```python
from build123d import *

# Parameters (mm, degrees)
BOSS_EXTRUDE1_DEPTH   = 9.525
FILLET1_R             = 5.08
F_5_0MM_DOWEL_HOLE1_D = 5
SKETCH14_R            = 2.5
CUT_EXTRUDE1_DEPTH    = 139.21913576


with BuildPart() as part:
    # Sketch1 → Boss-Extrude1 (new body)
    with BuildSketch(Plane.XY):
        Polygon((-27.510468203, 50), (27.510468203, 50), (67.924987047, 120), (67.924987047, 81.9), (20.64, 0), (10, -99.432340815), (-10, -99.432340815), (-20.64, 0), (-67.924987047, 81.9), (-67.924987047, 120), align=None)
    extrude(amount=BOSS_EXTRUDE1_DEPTH)

    # Fillet1
    fillet1_edges = [part.edges().sort_by_distance(p)[0] for p in [
        (-27.510468203, 50, 4.7625),
        (27.510468203, 50, 4.7625),
        (67.924987047, 81.9, 4.7625),
        (20.64, 0, 4.7625),
        (10, -99.432340815, 4.7625),
        (-10, -99.432340815, 4.7625),
        (-20.64, 0, 4.7625),
        (-67.924987047, 81.9, 4.7625),
    ]]
    fillet(fillet1_edges, radius=FILLET1_R)

    # Ø5.0mm Dowel Hole1 (through all)
    with Locations(Plane(origin=(0, 0, 0), x_dir=(-1, 0, 0), z_dir=(0, 0, -1))):
        with Locations((-7.5, 31.965654583), (7.5, 31.965654583), (-7.5, 16.965654583), (7.5, 16.965654583)):
            Hole(F_5_0MM_DOWEL_HOLE1_D / 2)

    # Sketch14 → Cut-Extrude1 (cut, through all)
    with BuildSketch(Plane.XY.offset(9.525)):
        with Locations((0, -89.432340815)):
            Circle(SKETCH14_R)
    extrude(amount=-CUT_EXTRUDE1_DEPTH, mode=Mode.SUBTRACT)


solid = part.part
```
CAD build for the part. Positions are in the model's coordinates, mm. A direction names the side the tool comes from. Coordinates: 2 decimals unless noted, no trailing zeros. Loops run counter-clockwise (first coordinate to the right, second up) from the corner with the lowest first, then second, coordinate; pieces in that order, holes last. Notation, with made-up numbers: (89, 33.5) - (143, 33.5) arc R20 cw to (143, 40.5) - close; hole circle Ø2 at (59.25, 63). An arc over 180 degrees is marked (long way). Return JSON: item names as keys, results as strings.
1. Probe L1, parallel to Y at x = 8, z = 3; L2, parallel to Y at x = 0, z = 7.25; L3, parallel to Y at x = -7.5, z = 3. List the from-to ranges inside material, lowest first. Write a range as from..to.
Result:
{"L1": "y = -98.74..14.52, 19.42..29.52, 34.42..50", "L2": "y = -99.43..-91.93, -86.93..50", "L3": "y = -98.99..14.47, 19.47..29.47, 34.47..50"}
2. Drop flat-ended pins along their axis: pin 1 (5 mm diameter, centred on x = -49.5, z = 3, fed in from -Y); pin 2 (4.5 mm diameter, centred on x = 0, y = -89.43, fed in from +Z); pin 3 (4 mm diameter, centred on x = 7, z = 4.5, fed in from +Y); pin 4 (5 mm diameter, centred on y = -43.5, z = 2, fed in from -X). Give the stop position or say it passes through.
Result:
{"pin 1": "stops at y = 45.66", "pin 2": "passes through", "pin 3": "stops at y = 50", "pin 4": "stops at x = -16.25"}
3. Band-saw the part on C-C (z = 2.25). Give the cut face in (x, y).
Result:
{"outline": "(-67.92, 83.26) arc R5.08 ccw to (-67.24, 80.72) - (-21.18, 0.93) arc R5.08 cw to (-20.53, -1.07) - (-10.49, -94.89) arc R5.08 ccw to (-5.43, -99.43) - (5.43, -99.43) arc R5.08 ccw to (10.49, -94.89) - (20.53, -1.07) arc R5.08 cw to (21.18, 0.93) - (67.24, 80.72) arc R5.08 ccw to (67.92, 83.26) - (67.92, 120) - (28.98, 52.54) arc R5.08 cw to (24.58, 50) - (-24.58, 50) arc R5.08 cw to (-28.98, 52.54) - (-67.92, 120) - close; hole circle Ø5 at (-7.5, 16.97); hole circle Ø5 at (-7.5, 31.97); hole circle Ø5 at (0, -89.43); hole circle Ø5 at (7.5, 16.97); hole circle Ø5 at (7.5, 31.97)"}
4. Band-saw the part on D-D (y = -35). Give the cut face in (x, z) (3 decimals).
Result:
{"outline": "(-16.895, 0) - (16.895, 0) - (16.895, 9.525) - (-16.895, 9.525) - close"}
5. Mould opens along X. For faces 3 (the cylindrical face through (8.654, 14.748, 4.829)), 4 (the cylindrical face through (8.869, -98.096, 4.829)), 5 (the flat face through (0, 11, 9.525)) say: released by +X, released by -X, zero draft, split by the parting line, or undercut.
Result:
{"face 3": "undercut", "face 4": "released by +X", "face 5": "zero draft"}
6. Band-saw the part on A-A (x = 0). Give the cut face in (y, z) (3 decimals).
Result:
{"outline": "(-99.432, 0) - (-91.932, 0) - (-91.932, 9.525) - (-99.432, 9.525) - close; (-86.932, 0) - (50, 0) - (50, 9.525) - (-86.932, 9.525) - close"}
7. 3-axis set-ups, long thin cutter, end or side, ignore diameter. For faces 1 (the cylindrical face through (-27.085, 50.662, 4.829)), 2 (the cylindrical face through (8.654, 29.748, 4.829)): which of +Z, -Z, +X, -X, +Y, -Y reach the whole face in a straight line?
Result:
{"face 1": "+Z, -Z, +Y", "face 2": "+Z, -Z"}
8. Band-saw the part on B-B (y = 96.5). Give the cut face in (x, z) (3 decimals), and give its area (3 significant figures).
Result:
{"outline": "(-67.925, 0) - (-54.357, 0) - (-54.357, 9.525) - (-67.925, 9.525) - close; (54.357, 0) - (67.925, 0) - (67.925, 9.525) - (54.357, 9.525) - close", "area": "258 mm2"}
